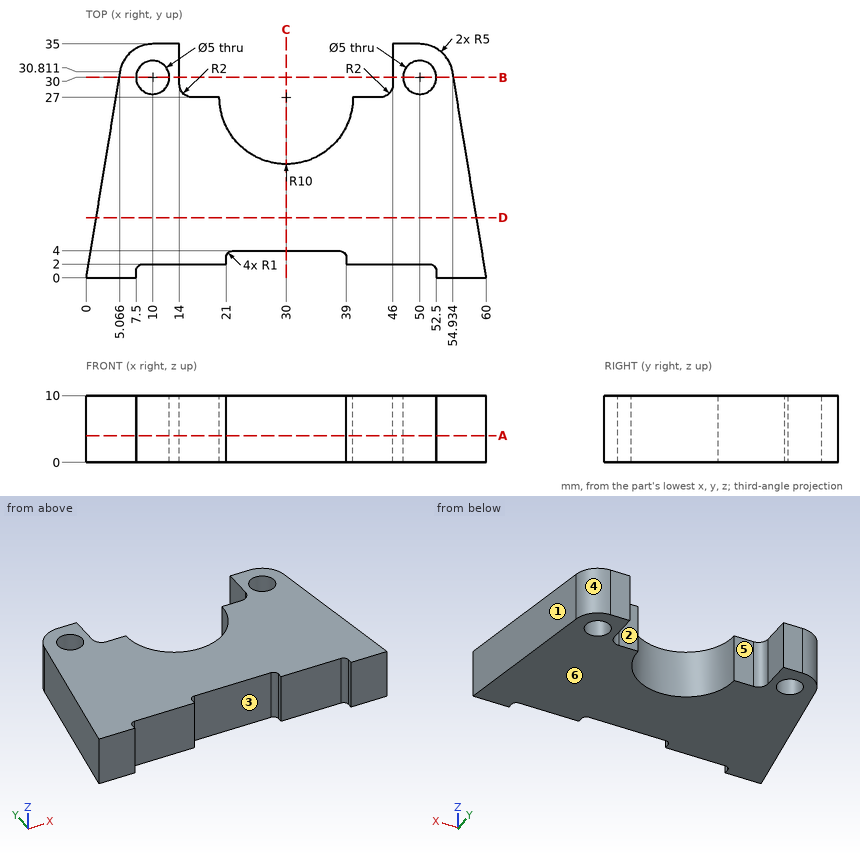
Job drawing, mm, ordinate dimensions from the low corner. One solid piece. A direction names the side the tool comes from. Coordinates: 2 decimals unless noted, no trailing zeros. Order: outer loops, then holes, each group sorted by start corner. A loop starts at its lowest first (then second) coordinate and runs counter-clockwise, first axis right, second up. Notation, with made-up numbers: (-29.5, -21.5) -> (5.5, -21.5) arc R24 cw to (5.5, 1.5) -> close; hole circle Ø8 at (31, 9). An arc over 180 degrees is marked (long way). Return JSON: item names as keys, results as strings. Group by question number.
Item 1: Wall check: line 1 along X through (y, z) = (29, 9); line 2 along Y through (x, z) = (10, 6); line 3 along Y through (x, z) = (48, 1). Give the ranges that are in metal, low to high. Write a range as [from, to].
Item 2: Tool access for the marked faces 1, 2 and 3: list every direction of +Z, -Z, +X, -X, +Y, -Y with a clear straight run to the whole face (end or side of a thin tool).
Item 3: Pull direction X, two halves, no side cores. Call the marked faces 4, 5 and 6: pulls with the +X half, pulls with the -X half, needs draft (parallel to the pull), parting line crosses it, or undercut.
Item 4: Saw through at C-C on x = 30. Write the cut outline in (y, z), then the cut area to 3 significant figures.
Item 5: Saw through at B-B on y = 30. Write the cut outline in (x, z).
Item 6: Saw through at D-D on y = 9. Write the cut outline in (x, z), then the cut area to 3 significant figures.
Item 7: Flat gauge pins, fed straight in: P1, Ø0.5, axis at y = 2.5, z = 7, coming from the +X side; P2, Ø5, axis at y = 33, z = 7.5, coming from the -X side (3 decimals); P3, Ø2, axis at y = 30.5, z = 3.5, coming from the +X side. Where does each tip first touch, or does it go through?
Item 8: Saw through at A-A on z = 4. Write the cut outline in (x, y), then the cut area to 3 significant figures.
Values found:
{
 "1": {"line 1": "x = [4.77, 7.71], [12.29, 14], [46, 47.71], [52.29, 55.23]", "line 2": "y = [2, 27.5], [32.5, 35]", "line 3": "y = [2, 28.5], [31.5, 35]"},
 "2": {"face 1": "+Z, -Z, +X, +Y", "face 2": "+Z, -Z, +Y", "face 3": "+Z, -Z, -Y"},
 "3": {"face 4": "pulls with the +X half", "face 5": "undercut", "face 6": "needs draft"},
 "4": {"outline": "(4, 0) -> (17, 0) -> (17, 10) -> (4, 10) -> close", "area": "130 mm2"},
 "5": {"outline": "(4.93, 0) -> (7.5, 0) -> (7.5, 10) -> (4.93, 10) -> close; (12.5, 0) -> (14, 0) -> (14, 10) -> (12.5, 10) -> close; (46, 0) -> (47.5, 0) -> (47.5, 10) -> (46, 10) -> close; (52.5, 0) -> (55.07, 0) -> (55.07, 10) -> (52.5, 10) -> close"},
 "6": {"outline": "(1.48, 0) -> (58.52, 0) -> (58.52, 10) -> (1.48, 10) -> close", "area": "570 mm2"},
 "7": {"P1": "stops at x = 59.63", "P2": "stops at x = 5.015", "P3": "stops at x = 55.15"},
 "8": {"outline": "(0, 0) -> (7.5, 0) -> (7.5, 1) arc R1 cw to (8.5, 2) -> (21, 2) -> (21, 3) arc R1 cw to (22, 4) -> (38, 4) arc R1 cw to (39, 3) -> (39, 2) -> (51.5, 2) arc R1 cw to (52.5, 1) -> (52.5, 0) -> (60, 0) -> (54.93, 30.81) arc R5 ccw to (50, 35) -> (46, 35) -> (46, 29) arc R2 cw to (44, 27) -> (40, 27) arc R10 cw to (20, 27) -> (16, 27) arc R2 cw to (14, 29) -> (14, 35) -> (10, 35) arc R5 ccw to (5.07, 30.81) -> close; hole circle Ø5 at (10, 30); hole circle Ø5 at (50, 30)", "area": "1,320 mm2"}
}
